The listing builds one solid part. Answer for the finished solid, in the listing's coordinates (mm). Coordinates: 2 decimals unless noted, no trailing zeros. Order: outer loops, then holes, each group sorted by start corner. A loop starts at its lowest first (then second) coordinate and runs counter-clockwise, first axis right, second up.
```python
from build123d import *

# Parameters (mm, degrees)
PAD047_DEPTH    = 4
POCKET007_DEPTH = 10
FILLET_R        = 1


with BuildPart() as part:
    # Sketch069 → Pad047 (new body)
    with BuildSketch(Plane.XY):
        Polygon((0, 10), (0, 0), (20, 0), align=None)
    extrude(amount=PAD047_DEPTH)

    # Sketch070 (on Face2 of Pad047) → Pocket007 (cut)
    with BuildSketch(Plane.XZ):
        Polygon((0, 4), (22.047997, 0), (22.047997, 4), align=None)
    extrude(amount=-POCKET007_DEPTH, mode=Mode.SUBTRACT)

    # Fillet
    fillet_edges = [part.edges().sort_by_distance(p)[0] for p in [
        (10, 0, 2.185776),
    ]]
    fillet(fillet_edges, radius=FILLET_R)


solid = part.part
```
(1) Find section B-B (y = 2.25). Write down the section's boundary in (x, z).
(2) This flat-tipped pin is pushed along its axis until it touches: pin 1 Ø1 at (x, y) = (11.5, 6.5) entering from -Z. Where does it stop, or does it pass through?
(3) Consider line 1 (X direction, y = 1, z = 0.3); line 2 (X direction, y = 8, z = 2.5); line 3 (Z direction, x = 10, y = 4.25). Determine where each line is inside the solid, lowest interval first.
(4) Find section A-A (y = 6.25). Write down the section's boundary in (x, z).
Findings below:
1. outline: (0, 0) - (15.5, 0) - (15.5, 1.19) - (0, 4) - close
2. pin 1: passes through
3. line 1: x = 0 to 18
3. line 2: x = 0 to 4
3. line 3: z = 0 to 2.19
4. outline: (0, 0) - (7.5, 0) - (7.5, 2.64) - (0, 4) - close
